Design review of the part built by this model. Coordinates are the model's own, in mm. Coordinates: 2 decimals unless noted, no trailing zeros. Write each loop counter-clockwise with the first axis right and the second up, starting at its lowest first coordinate (ties: lowest second). Pieces come first, ordered by that corner, then holes.
Q1. Add section D-D, the plane z = 8. Give the boundary of the cut face in (x, y), plus the area to 3 significant figures.
Q2. Add section C-C, the plane z = 10.25. Give the boundary of the cut face in (x, y), plus the area to 3 significant figures.
Q3. The part is to be moulded in two halves that separate along Y. For faces 1 (the face through (-1.591, -7.165, 13.26)), 2 (the face through (-0.2, 3.3, 0)), 3 (the face through (3.24, -2.485, 6.558)), say which applies: +Y half, -Y half, draft (parallel to the pull), parting line (faces both ways), or undercut.
Q4. Clearance check with flat-ended pins moving along their axes: pin 1 Ø2 at (y, z) = (-8, 4) entering from +X; pin 2 Ø1 at (x, y) = (-1.5, 5) entering from +Z; pin 3 Ø1 at (y, z) = (-4.5, 4) entering from +X. State where each tip first meets the part, or that it passes through.
Q5. Add section A-A, the plane y = 0. Give the boundary of the cut face in (x, z).
Q6. To check wall thickness, follow probe 1 along Y at (x, z) = (0, 1.95); probe 2 along Y at (x, z) = (-3, 6.25); probe 3 along X at (y, z) = (-4, 9.75). State the ranges of each line that lie inside material, in increasing order.
from build123d import *

# Parameters (mm, degrees)
F0_R           = 14
F1_DEPTH       = 14.6
F3_SIZE        = 8
F4_D           = 6
F4_START       = 1
F4_CSINK_D     = 14
F4_CSINK_ANGLE = 45


with BuildPart() as f1:
    # F0 (on Top) → F1 (new body)
    with BuildSketch(Plane.XY):
        Circle(F0_R)
    extrude(amount=F1_DEPTH)

    # F3
    f3_edges = [f1.edges().sort_by_distance(p)[0] for p in [
        (-14, 0, 14.6),
    ]]
    chamfer(f3_edges, length=F3_SIZE)

    # F4 (through all)
    # its depths count from where the whole tool has entered the part; down to there all is cleared
    with Locations(Plane.XY.offset(14.6).offset(-F4_START)):
        with Locations((0, 0)):
            CounterSinkHole(F4_D / 2, F4_CSINK_D / 2, counter_sink_angle=F4_CSINK_ANGLE)


solid = f1.part
Here are the results:
1. outline: circle Ø25.2 at (0, 0); hole circle Ø9.36 at (0, 0)
1. area: 430 mm2
2. outline: circle Ø20.7 at (0, 0); hole circle Ø11.22 at (0, 0)
2. area: 238 mm2
3. face 1: parting line
3. face 2: draft
3. face 3: undercut
4. pin 1: stops at x = 12.12
4. pin 2: stops at z = 10.51
4. pin 3: stops at x = 13.42
5. outline: (-14, 0) - (-3, 0) - (-3, 3.94) - (-7, 13.6) - (-14, 6.6) - close; (3, 0) - (14, 0) - (14, 6.6) - (7, 13.6) - (3, 3.94) - close
6. probe 1: y = -14 to -3, 3 to 14
6. probe 2: y = -13.67 to -2.58, 2.58 to 13.67
6. probe 3: x = -10.09 to -3.64, 3.64 to 10.09
